Here's how the part is built. I have some questions about the finished solid (model axes, mm). A direction names the side the tool comes from. Give positions to 0.01 mm unless a question says otherwise; leave off trailing zeros. Loops run counter-clockwise (first coordinate to the right, second up) from the corner with the lowest first, then second, coordinate; pieces in that order, holes last.
Q1. For faces 5 (the face through (-20.305, -13.218, -16.731)), 6 (the face through (-5, -12.817, -11)), which set-ups out of +Z, -Z, +X, -X, +Y, -Y let a thin tool reach every point of the face, with its end or its side?
Q2. If we section it at C-C (x = -7): Please give me the cut outline in (y, z) (1 decimal), plus the area to 3 significant figures.
Q3. We'd pull the mould along Z, two halves only. Please class faces 1 (the face through (-5.96, 4.18, -16.73)), 2 (the face through (-5.96, -13.22, -16.73)), 3 (the face through (-17.18, -1.43, 0.4)), 4 (the face through (-5.77, 3.32, -0.48)): +Z half, -Z half, draft (parallel to the pull), parting line (faces both ways), or undercut.
Q4. Will these pins go through, and if not, where does the flat tip stop? P1, Ø3, axis at x = -16.65, y = -2.27, coming from the +Z side; P2, Ø1.8, axis at x = -9.68, y = -6.82, coming from the -Z side; P3, Ø3, axis at x = 2.5, y = -3, coming from the -Z side.
Q5. If we section it at B-B (y = -1.75): Please give me the cut outline in (x, z).
Q6. I need wall thicknesses on line 1 (Y direction, x = -2, z = -3.25); line 2 (Z direction, x = -14, y = -0.5); line 3 (Y direction, x = -14, z = -0.5). Which ranges of each line are inside material? Lowest first, please.
Q7. If we section it at A-A (z = -10.5): Please give me the cut outline in (x, y), plus the area to 3 significant figures.
Q8. If we section it at D-D (y = -9.5): Please give me the cut outline in (x, z).
from build123d import *

# Parameters (mm, degrees)
BASE_FLANGE1_DEPTH              = 0.8128
EDGE_FLANGE1_STRIP_W            = 6.4262
EDGE_FLANGE1_STRIP_H            = 0.8128
EDGE_FLANGE1_STRIP_CUT_DEPTH    = 35.042145822
EDGE_FLANGE1_STRIP_2_W          = 6.4262
EDGE_FLANGE1_STRIP_2_H          = 0.8128
EDGE_FLANGE1_STRIP_CUT_2_DEPTH  = 35.042145822
EDGE_FLANGE1_DEPTH              = 35.042145822
EDGE_FLANGE1_BEND_DEPTH         = 35.042145822
F_1_8_0_125_DIAMETER_HOLE1_D    = 3.175
F_56_0_0465_DIAMETER_HOLE1_D    = 1.1811
F_5_64_0_07813_DIAMETER_HOLE1_D = 1.984502


# Sheet-metal steps are written as plain solids
with BuildPart() as part:
    # Sketch1 → Base-Flange1 (new body)
    with BuildSketch(Plane.XY):
        Polygon((-23.044963434, -12.817151558), (5.647182388, -12.817151558), (11.997182388, -12.817151558), (11.997182388, 3.772848442), (5.647182388, 3.772848442), (-23.044963434, 3.772848442), align=None)
    extrude(amount=BASE_FLANGE1_DEPTH)

    # Edge-Flange1 strip (across the edge) → Edge-Flange1 strip cut (cut)
    with BuildSketch(Plane(origin=(-23.044963434, 3.772848442, 0), x_dir=(0, -1, 0), z_dir=(1, 0, 0))):
        with Locations((-1.6256, -0.4064)):
            Rectangle(EDGE_FLANGE1_STRIP_W, EDGE_FLANGE1_STRIP_H)
    extrude(amount=EDGE_FLANGE1_STRIP_CUT_DEPTH, mode=Mode.SUBTRACT)

    # Edge-Flange1 strip 2 (across the edge) → Edge-Flange1 strip cut 2 (cut)
    with BuildSketch(Plane(origin=(11.997182388, -12.817151558, 0), x_dir=(0, 1, 0), z_dir=(-1, 0, 0))):
        with Locations((-1.6256, -0.4064)):
            Rectangle(EDGE_FLANGE1_STRIP_2_W, EDGE_FLANGE1_STRIP_2_H)
    extrude(amount=EDGE_FLANGE1_STRIP_CUT_2_DEPTH, mode=Mode.SUBTRACT)

    # Edge-Flange1 section (across the edge) → Edge-Flange1 (add)
    with BuildSketch(Plane(origin=(-23.044963434, 3.772848442, 0), x_dir=(0, -1, 0), z_dir=(1, 0, 0))):
        with BuildLine():
            Line((-0.8128, 1.5875), (-0.8128, 19.5072))
            Line((-0.8128, 19.5072), (0, 19.5072))
            Line((0, 19.5072), (0, 1.5875))
            ThreePointArc((0, 1.5875), (0.464967985, 0.464967985), (1.5875, 0))
            Line((1.5875, 0), (1.5875, -0.8128))
            ThreePointArc((1.5875, -0.8128), (-0.109768407, -0.109768407), (-0.8128, 1.5875))
        make_face()
    extrude(amount=EDGE_FLANGE1_DEPTH)

    # Edge-Flange1 section 2 (across the edge) → Edge-Flange1 bend (add)
    with BuildSketch(Plane(origin=(11.997182388, -12.817151558, 0), x_dir=(0, 1, 0), z_dir=(-1, 0, 0))):
        with BuildLine():
            Line((-0.8128, 1.5875), (-0.8128, 19.5072))
            Line((-0.8128, 19.5072), (0, 19.5072))
            Line((0, 19.5072), (0, 1.5875))
            ThreePointArc((0, 1.5875), (0.464967985, 0.464967985), (1.5875, 0))
            Line((1.5875, 0), (1.5875, -0.8128))
            ThreePointArc((1.5875, -0.8128), (-0.109768407, -0.109768407), (-0.8128, 1.5875))
        make_face()
    extrude(amount=EDGE_FLANGE1_BEND_DEPTH)

    # 1/8 (0.125) Diameter Hole1 (through all)
    with Locations(Plane(origin=(0, -13.629951558, 0), x_dir=(-1, 0, 0), z_dir=(0, -1, 0))):
        with Locations((-5.647182388, 16.3322)):
            Hole(F_1_8_0_125_DIAMETER_HOLE1_D / 2)

    # #56 (0.0465) Diameter Hole1 (through all)
    with Locations(Plane(origin=(0, -13.629951558, 0), x_dir=(-1, 0, 0), z_dir=(0, -1, 0))):
        with Locations((5.523890523, 16.3322), (19.869963434, 16.3322), (19.869963434, 4.7625), (-8.822182388, 4.7625)):
            Hole(F_56_0_0465_DIAMETER_HOLE1_D / 2)

    # 5/64 (0.07813) Diameter Hole1 (through all)
    with Locations(Plane.XY.offset(0.8128)):
        with Locations((-16.648897162, -2.269651558), (-9.683897162, -6.824651558)):
            Hole(F_5_64_0_07813_DIAMETER_HOLE1_D / 2)


solid = part.part
Check sheet entries:
1. face 5: +Y, -Y
1. face 6: -Z, +X, -X
2. outline: (-13.6, -19.5) - (-12.8, -19.5) - (-12.8, -1.6) arc R1.6 cw to (-11.2, 0) - (2.2, 0) arc R1.6 cw to (3.8, -1.6) - (3.8, -19.5) - (4.6, -19.5) - (4.6, -1.6) arc R2.4 ccw to (2.2, 0.8) - (-11.2, 0.8) arc R2.4 ccw to (-13.6, -1.6) - close
2. area: 45.1 mm2
3. face 1: undercut
3. face 2: undercut
3. face 3: draft
3. face 4: -Z half
4. P1: stops at z = 0.81
4. P2: passes through
4. P3: stops at z = 0
5. outline: (-23.04, 0) - (-17.49, 0) - (-17.49, 0.81) - (-23.04, 0.81) - close; (-15.8, 0) - (12, 0) - (12, 0.81) - (-15.8, 0.81) - close
6. line 1: y = -13.63 to -12.82, 3.77 to 4.59
6. line 2: z = 0 to 0.81
6. line 3: y = -13.37 to -12.39, 3.34 to 4.33
7. outline: (-23.04, -13.63) - (12, -13.63) - (12, -12.82) - (-23.04, -12.82) - close; (-23.04, 3.77) - (12, 3.77) - (12, 4.59) - (-23.04, 4.59) - close
7. area: 57.0 mm2
8. outline: (-23.04, 0) - (12, 0) - (12, 0.81) - (-23.04, 0.81) - close
